Input: part model. Units: mm. Frame: model coordinates. Face numbers are marked on the shaded views. A direction names the side the tool comes from. Round coordinates to 2 decimals unless told otherwise and drop trailing zeros. Loops run counter-clockwise (first coordinate to the right, second up) from the corner with the lowest first, then second, coordinate; pieces in that order, holes last. Notation, with made-up numbers: (-16.75, 59) - (13.25, 59) arc R32 ccw to (13.25, 92) - close; hole circle Ø1 at (67.5, -0.5). An arc over 180 degrees is marked (long way). Write each question's results on one line, items separated by ' | '.
from build123d import *

# Parameters (mm, degrees)
SKETCH1_W               = 25.3746
SKETCH1_H               = 25.3746
BOSS_EXTRUDE1_DEPTH     = 12.6873
SKETCH2_OUTSIDE_W       = 127.528
SKETCH2_OUTSIDE_H       = 127.528
SKETCH2_OUTSIDE_R       = 12.6873
CUT_EXTRUDE1_DEPTH      = 26.3746
CUT_EXTRUDE1_TAPER      = 60
SKETCH3_R               = 4.7625
CUT_EXTRUDE2_DEPTH      = 13.6873
CUT_EXTRUDE2_DEPTH_BACK = 13.6873
SKETCH3_2_R             = 4.7625
BOSS_EXTRUDE3_DEPTH     = 19.05
CHAMFER6_SIZE           = 1.27


with BuildPart() as part:
    # Sketch1 → Boss-Extrude1 (new body, symmetric)
    with BuildSketch(Plane.XY):
        Rectangle(SKETCH1_W, SKETCH1_H)
    extrude(amount=BOSS_EXTRUDE1_DEPTH, both=True)

    # Sketch2 outside → Cut-Extrude1 (cut, through all)
    with BuildSketch(Plane(origin=(12.6873, 0, 0), x_dir=(0, 0, -1), z_dir=(1, 0, 0))):
        Rectangle(SKETCH2_OUTSIDE_W, SKETCH2_OUTSIDE_H)
        Circle(SKETCH2_OUTSIDE_R, mode=Mode.SUBTRACT)
    cut_extrude1 = extrude(amount=-CUT_EXTRUDE1_DEPTH, taper=CUT_EXTRUDE1_TAPER, mode=Mode.SUBTRACT)

    # Mirror1: Cut-Extrude1 across plane
    add(cut_extrude1.mirror(Plane(origin=(0, 0, 0), x_dir=(0, 0, 1), z_dir=(1, 0, 0))), mode=Mode.SUBTRACT)

    # Sketch3 → Cut-Extrude2 (cut, two sides)
    with BuildSketch(Plane.XY) as cut_extrude2_sk:
        Circle(SKETCH3_R)
    extrude(amount=CUT_EXTRUDE2_DEPTH, mode=Mode.SUBTRACT)
    extrude(cut_extrude2_sk.sketch, amount=-CUT_EXTRUDE2_DEPTH_BACK, mode=Mode.SUBTRACT)

    # Sketch3<2> → Boss-Extrude3 (add, symmetric)
    with BuildSketch(Plane.XY):
        Circle(SKETCH3_2_R)
    boss_extrude3 = extrude(amount=BOSS_EXTRUDE3_DEPTH, both=True)

    # Mirror2: Boss-Extrude3 across plane
    add(boss_extrude3.mirror(Plane(origin=(0, 0, 0), x_dir=(-0.707106781, 0, 0.707106781), z_dir=(-0.707106781, 0, -0.707106781))))

    # Chamfer6
    chamfer6_edges = [part.edges().sort_by_distance(p)[0] for p in [
        (-4.7625, 0, -19.05),
        (-4.7625, 0, 19.05),
        (-19.05, 0, 4.7625),
        (19.05, 0, 4.7625),
    ]]
    chamfer(chamfer6_edges, length=CHAMFER6_SIZE)


solid = part.part
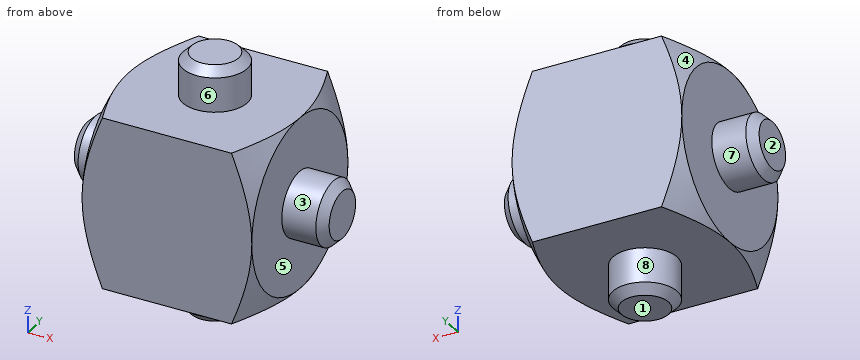
1. Mould query, pull axis Z, two halves, no side actions, for the marked faces 1, 2, 3 and 4. Classes: pulls with the +Z half, pulls with the -Z half, needs draft (parallel to the pull), parting line crosses it, or undercut.
Answer:
face 1: pulls with the -Z half | face 2: needs draft | face 3: parting line crosses it | face 4: pulls with the +Z half
2. Set-up query: the marked faces 5, 6, 7 and 8. Return all of +Z, -Z, +X, -X, +Y, -Y with unobstructed straight access to the full face (end or side cutting, diameter ignored); none if empty.
Answer:
face 5: +X | face 6: +Z | face 7: -X | face 8: -Z
3. Contact query for flat-ended pins moving along their axis: pin 1 (6 mm diameter, centred on x = -13.5, y = 5, fed in from -Z); pin 2 (1.5 mm diameter, centred on y = 4, z = 6, fed in from -X); pin 3 (1.5 mm diameter, centred on x = 4, y = -7.5, fed in from +Z). Output: stop coordinate, or through.
Answer:
pin 1: z = -12.69 | pin 2: x = -12.69 | pin 3: z = 12.69
4. Section query B-B, the plane z = -15. Output: boundary loops of the cut face in (x, y) (1 decimal).
Answer:
outline: circle Ø9.5 at (0, 0)
5. Section query A-A, the plane x = 0. Output: boundary loops of the cut face in (y, z), plus the area to 3 significant figures.
Answer:
outline: (-12.69, -12.69) - (-4.76, -12.69) - (-4.76, -17.78) - (-3.49, -19.05) - (3.49, -19.05) - (4.76, -17.78) - (4.76, -12.69) - (12.69, -12.69) - (12.69, 12.69) - (4.76, 12.69) - (4.76, 17.78) - (3.49, 19.05) - (-3.49, 19.05) - (-4.76, 17.78) - (-4.76, 12.69) - (-12.69, 12.69) - close | area: 762 mm^2
6. Line query: line 1 (X direction, y = 7.5, z = 1.5); line 2 (Z direction, x = -13, y = -0.25). Output: solid intervals per line, ascending. Write a range as [from, to].
Answer:
line 1: [-12.69, 12.69] | line 2: [-4.76, 4.76]
